Design review of the part built by this model. Coordinates are the model's own, in mm. Face numbers are marked on the shaded views. Coordinates: 2 decimals unless noted, no trailing zeros. Loops run counter-clockwise (first coordinate to the right, second up) from the corner with the lowest first, then second, coordinate; pieces in that order, holes last. Notation, with made-up numbers: (64.25, 83.5) -> (104.25, 83.5) arc R31 ccw to (104.25, 111.5) -> close; hole circle Ø1 at (-31, 6.5). An arc over 180 degrees is marked (long way). Answer as a JSON object with one key per item and string values.
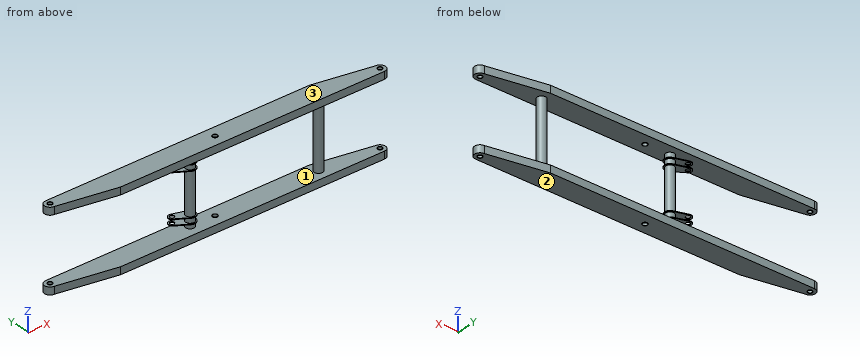
```python
from build123d import *

# Parameters (mm, degrees)
EXTRUDE_1_DEPTH        = 100
SKETCH_2_R             = 30
CUT_EXTRUDE_1_DEPTH    = 100
SKETCH_3_R             = 32.5
SKETCH_3_R_2           = 30
EXTRUDE_2_DEPTH        = 5
EXTRUDE_START          = 5
SKETCH_4_R             = 32.5
SKETCH_4_R_2           = 30
EXTRUDE_3_DEPTH        = 5
SKETCH_5_R             = 30
CUT_EXTRUDE_3_DEPTH    = 552
SKETCH_6_R             = 35
SKETCH_6_R_2           = 30
EXTRUDE_4_DEPTH        = 5
SKETCH_7_R             = 35
SKETCH_7_R_2           = 30
EXTRUDE_5_DEPTH        = 5
SKETCH_8_R             = 60
EXTRUDE_6_DEPTH        = 448
SKETCH_9_R             = 60
EXTRUDE_7_DEPTH        = 896
EXTRUDE_8_DEPTH        = 10
EXTRUDE_10_DEPTH       = 10
CUT_EXTRUDE_START      = -10
CUT_EXTRUDE_6_DEPTH    = 10
PATTERN_LINEAR_2_COUNT = 2
PATTERN_LINEAR_2_PITCH = 80
SKETCH_16_R            = 30
CUT_EXTRUDE_7_DEPTH    = 95
MIRROR_START           = -160
MIRROR_3_OUTLINE_R     = 30
MIRROR_3_DEPTH         = 10
MIRROR_START_2         = -80
MIRROR_3_2_OUTLINE_R   = 30
MIRROR_3_2_DEPTH       = 10
SCALE1_SCALE           = 0.345


# Read off the part's stored shape, not the designer's step: 镜向3
with BuildPart() as part:
    # 草图1 → 凸台-拉伸1 (new body)
    with BuildSketch(Plane.XY):
        with BuildLine():
            Line((-60.1323511, -127.533248731), (739.8676489, -277.533248731))
            Line((739.8676489, -277.533248731), (4439.8676489, -277.533248731))
            ThreePointArc((4439.8676489, -277.533248731), (4514.8676489, -202.533248731), (4439.8676489, -127.533248731))
            Line((4439.8676489, -127.533248731), (3639.8676489, 22.466751269))
            Line((3639.8676489, 22.466751269), (-60.1323511, 22.466751269))
            ThreePointArc((-60.1323511, 22.466751269), (-135.1323511, -52.533248731), (-60.1323511, -127.533248731))
        make_face()
    extrude(amount=EXTRUDE_1_DEPTH)

    # 草图2 → 切除-拉伸1 (cut)
    with BuildSketch(Plane.XY.offset(100)):
        with Locations((-60.1323511, -52.533248731)):
            Circle(SKETCH_2_R)
        with Locations((4439.8676489, -202.533248731)):
            Circle(SKETCH_2_R)
    extrude(amount=-CUT_EXTRUDE_1_DEPTH, mode=Mode.SUBTRACT)

    # 草图3 → 凸台-拉伸2 (add)
    # profile 1 of 2: a face of its own
    with BuildSketch(Plane(origin=(0, 0, 0), x_dir=(-1, 0, 0), z_dir=(0, 0, -1))):
        with Locations(Location((-4439.8676489, -202.533248731, 0), (0, 0, 180))):
            Circle(SKETCH_3_R)
        with Locations(Location((-4439.8676489, -202.533248731, 0), (0, 0, 180))):
            Circle(SKETCH_3_R_2, mode=Mode.SUBTRACT)
    # profile 2 of 2: a face of its own
    with BuildSketch(Plane(origin=(0, 0, 0), x_dir=(-1, 0, 0), z_dir=(0, 0, -1))):
        with Locations(Location((60.1323511, -52.533248731, 0), (0, 0, 180))):
            Circle(SKETCH_3_R)
        with Locations(Location((60.1323511, -52.533248731, 0), (0, 0, 180))):
            Circle(SKETCH_3_R_2, mode=Mode.SUBTRACT)
    extrude(amount=EXTRUDE_2_DEPTH)

    # 草图4 → 凸台-拉伸3 (add)
    # profile 1 of 2: a face of its own
    with BuildSketch(Plane.XY.offset(100).offset(EXTRUDE_START)):
        with Locations((-60.1323511, -52.533248731)):
            Circle(SKETCH_4_R)
        with Locations((-60.1323511, -52.533248731)):
            Circle(SKETCH_4_R_2, mode=Mode.SUBTRACT)
    # profile 2 of 2: a face of its own
    with BuildSketch(Plane.XY.offset(100).offset(EXTRUDE_START)):
        with Locations((4439.8676489, -202.533248731)):
            Circle(SKETCH_4_R)
        with Locations((4439.8676489, -202.533248731)):
            Circle(SKETCH_4_R_2, mode=Mode.SUBTRACT)
    extrude(amount=-EXTRUDE_3_DEPTH)

    # 草图5 → 切除-拉伸3 (cut)
    with BuildSketch(Plane(origin=(0, 0, 0), x_dir=(-1, 0, 0), z_dir=(0, 0, -1))):
        with Locations((-2189.8676489, -127.533248731)):
            Circle(SKETCH_5_R)
    extrude(amount=-CUT_EXTRUDE_3_DEPTH, mode=Mode.SUBTRACT)

    # 草图6 → 凸台-拉伸4 (add)
    with BuildSketch(Plane.XY.offset(100)):
        with Locations((2189.8676489, -127.533248731)):
            Circle(SKETCH_6_R)
        with Locations(Location((2189.8676489, -127.533248731, 0), (0, 0, 180))):
            Circle(SKETCH_6_R_2, mode=Mode.SUBTRACT)
    extrude(amount=EXTRUDE_4_DEPTH)

    # 草图7 → 凸台-拉伸5 (add)
    with BuildSketch(Plane(origin=(0, 0, 0), x_dir=(-1, 0, 0), z_dir=(0, 0, -1)).offset(EXTRUDE_START)):
        with Locations(Location((-2189.8676489, -127.533248731, 0), (0, 0, 180))):
            Circle(SKETCH_7_R)
        with Locations((-2189.8676489, -127.533248731)):
            Circle(SKETCH_7_R_2, mode=Mode.SUBTRACT)
    extrude(amount=-EXTRUDE_5_DEPTH)

    # 草图8 → 凸台-拉伸6 (add)
    with BuildSketch(Plane(origin=(0, 0, 0), x_dir=(-1, 0, 0), z_dir=(0, 0, -1))):
        with Locations(Location((-3639.8676489, -127.533248731, 0), (0, 0, 180))):
            Circle(SKETCH_8_R)
    extrude(amount=EXTRUDE_6_DEPTH)

    # 镜向1: part across plane


with BuildPart() as part_1:
    add(part.part)
    add(part.part.mirror(Plane(origin=(3639.8676489, -127.533248731, -448), x_dir=(1, 0, 0), z_dir=(0, 0, -1))))

    # 草图9 → 凸台-拉伸7 (add)
    with BuildSketch(Plane.XY.offset(-896)):
        with Locations(Location((1839.8676489, -127.533248731, 0), (0, 0, 180))):
            Circle(SKETCH_9_R)
    extrude(amount=EXTRUDE_7_DEPTH)

    # 草图10 → 凸台-拉伸8 (add)
    with BuildSketch(Plane.XY.offset(-896)):
        with BuildLine():
            Line((1631.976489947, -85.328201293), (1799.923246582, -191.011156096))
            ThreePointArc((1799.923246582, -191.011156096), (1907.840732928, -159.229618362), (1862.818780211, -56.131248958))
            Line((1862.818780211, -56.131248958), (1673.9068457, 4.591736799))
            ThreePointArc((1673.9068457, 4.591736799), (1613.290702141, -21.878683296), (1631.976489947, -85.328201293))
        make_face()
    extrude(amount=EXTRUDE_8_DEPTH)

    # 草图14 → 凸台-拉伸10 (add)
    with BuildSketch(Plane.XY.offset(-826)):
        with BuildLine():
            Line((1631.976489947, -85.328201293), (1799.923246582, -191.011156096))
            ThreePointArc((1799.923246582, -191.011156096), (1907.840732928, -159.229618362), (1862.818780211, -56.131248958))
            Line((1862.818780211, -56.131248958), (1673.9068457, 4.591736799))
            ThreePointArc((1673.9068457, 4.591736799), (1613.290702141, -21.878683296), (1631.976489947, -85.328201293))
        make_face()
    extrude_10 = extrude(amount=EXTRUDE_10_DEPTH)

    # 草图15 → 切除-拉伸6 (cut)
    with BuildSketch(Plane.XY.offset(-886).offset(CUT_EXTRUDE_START)):
        with BuildLine():
            Line((1631.976489947, -85.328201293), (1799.923246582, -191.011156096))
            ThreePointArc((1799.923246582, -191.011156096), (1907.840732928, -159.229618362), (1862.818780211, -56.131248958))
            Line((1862.818780211, -56.131248958), (1673.9068457, 4.591736799))
            ThreePointArc((1673.9068457, 4.591736799), (1613.290702141, -21.878683296), (1631.976489947, -85.328201293))
        make_face()
    extrude(amount=CUT_EXTRUDE_6_DEPTH, mode=Mode.SUBTRACT)

    # 阵列(线性)2: 凸台-拉伸10 ×2
    with Locations(*[(0, 0, i * PATTERN_LINEAR_2_PITCH) for i in range(1, PATTERN_LINEAR_2_COUNT)]):
        add(extrude_10)

    # 草图16 → 切除-拉伸7 (cut)
    with BuildSketch(Plane.XY.offset(-736)):
        with Locations((1658.606091493, -43.009596383)):
            Circle(SKETCH_16_R)
    extrude(amount=-CUT_EXTRUDE_7_DEPTH, mode=Mode.SUBTRACT)

    # 镜向3 outline → 镜向3 (add)
    with BuildSketch(Plane.XY.offset(MIRROR_START)):
        with BuildLine():
            Line((1862.818780211, -56.131248958), (1673.9068457, 4.591736799))
            ThreePointArc((1673.9068457, 4.591736799), (1613.290702141, -21.878683296), (1631.976489947, -85.328201293))
            Line((1631.976489947, -85.328201293), (1799.923246582, -191.011156096))
            ThreePointArc((1799.923246582, -191.011156096), (1907.840732928, -159.229618361), (1862.818780211, -56.131248958))
        make_face()
        with Locations((1658.606091493, -43.009596383)):
            Circle(MIRROR_3_OUTLINE_R, mode=Mode.SUBTRACT)
    extrude(amount=MIRROR_3_DEPTH)

    # Mirror 3 2 outline → Mirror 3 2 (add)
    with BuildSketch(Plane.XY.offset(MIRROR_START_2)):
        with BuildLine():
            Line((1862.818780211, -56.131248958), (1673.9068457, 4.591736799))
            ThreePointArc((1673.9068457, 4.591736799), (1613.290702141, -21.878683296), (1631.976489947, -85.328201293))
            Line((1631.976489947, -85.328201293), (1799.923246582, -191.011156096))
            ThreePointArc((1799.923246582, -191.011156096), (1907.840732928, -159.229618361), (1862.818780211, -56.131248958))
        make_face()
        with Locations((1658.606091493, -43.009596383)):
            Circle(MIRROR_3_2_OUTLINE_R, mode=Mode.SUBTRACT)
    extrude(amount=MIRROR_3_2_DEPTH)


with BuildPart() as part_2:
    # Scale1: scaled about (2229.895561812, -127.384045127, -447.813736157)
    add(part_1.part.scale(SCALE1_SCALE).moved(Location((1460.581592987, -83.436549558, -293.317997183))))


solid = part_2.part
```
1) The part is to be moulded in two halves that separate along Z. For the marked faces 1, 2 and 3, say which applies: pulls with the +Z half, pulls with the -Z half, needs draft (parallel to the pull), parting line crosses it, or undercut.
Completed:
{"face 1": "undercut", "face 2": "pulls with the -Z half", "face 3": "pulls with the +Z half"}
2) Add section A-A, the plane x = 2526.5. Give the boundary of the cut face in (y, z), and give its area (3 significant figures).
Completed:
{"outline": "(-179.19, -636.94) -> (-75.69, -636.94) -> (-75.69, -602.44) -> (-179.19, -602.44) -> close; (-179.19, -293.32) -> (-75.69, -293.32) -> (-75.69, -258.82) -> (-179.19, -258.82) -> close", "area": "7,140 mm²"}
3) Add section C-C, the plane x = 1658.5. Give the boundary of the cut face in (y, z).
Completed:
{"outline": "(-168.44, -636.94) -> (-75.69, -636.94) -> (-75.69, -602.44) -> (-168.44, -602.44) -> close; (-168.44, -293.32) -> (-75.69, -293.32) -> (-75.69, -258.82) -> (-168.44, -258.82) -> close"}
4) Add section B-B, the plane z = -491.5. Give the boundary of the cut face in (x, y).
Completed:
{"outline": "circle Ø41.4 at (2095.34, -127.44); circle Ø41.4 at (2716.34, -127.44)"}
5) Clearance check with flat-ended pins moving along their axes: pin 1 Ø21.5 at (x, y) = (2083.5, -129.5) entering from +Z; pin 2 Ø16.5 at (x, y) = (1439.84, -101.56) entering from +Z; pin 3 Ø3 at (x, y) = (2457.5, -141.5) entering from -Z. State where each tip first meets the part, or that it passes through.
Completed:
{"pin 1": "z = -258.82", "pin 2": "through", "pin 3": "z = -636.94"}
6) Wall thickness on probe 1 along Z at (x, y) = (2726, -163.5); probe 2 along X at (y, z) = (-130, -579); probe 3 along X at (y, z) = (-124, -307): over which ranges is each line inside the solid? List them lowest first.
Completed:
{"probe 1": "-636.94 to -602.44, -293.32 to -258.82", "probe 2": "2074.8 to 2115.88, 2695.8 to 2736.88", "probe 3": "2074.92 to 2115.75, 2695.92 to 2736.75"}
